Check sheet for the modelled part. Datum: model origin and axes. Units: mm. A direction names the side the tool comes from. Round coordinates to 2 decimals unless told otherwise and drop trailing zeros. Write each loop counter-clockwise with the first axis right and the second up, starting at its lowest first coordinate (ties: lowest second). Pieces come first, ordered by that corner, then holes. Notation, with made-up numbers: M 76.25,48 L 130.25,48 A29 ccw 130.25,72 Z; hole C 68.25,86 d1. An arc over 180 degrees is marked long. Answer in a Markdown table with one row per item.
```python
from build123d import *

# Parameters (mm, degrees)
BASPROSKE_W             = 19.05
BASPROSKE_H             = 19.957142857
TOOTHCUT_DEPTH          = 35.051102802
TEETHCUTS_COUNT         = 20
BORSKE_R                = 6.35
BORE_DEPTH              = 50.8000508
KEYSKE_W                = 3.175
KEYSKE_H                = 7.4676
KEYWAY_DEPTH            = 50.8000508
SKETCH1_W               = 3.175
SKETCH1_H               = 0.4064
CUT_EXTRUDE4_DEPTH      = 34.838053031
CUT_EXTRUDE4_DEPTH_BACK = 34.838053031


with BuildPart() as part:
    # BasProSke → Base-Revolve (revolve)
    with BuildSketch(Plane(origin=(0, 0, 0), x_dir=(1, 0, 0), z_dir=(0, 1, 0)), mode=Mode.PRIVATE) as base_revolve_sk:
        with Locations((9.525, 9.978571429)):
            Rectangle(BASPROSKE_W, BASPROSKE_H)
    revolve(base_revolve_sk.sketch.rotate(Axis((-10, 0, 0), (1, 0, 0)), 180), axis=Axis((-10, 0, 0), (1, 0, 0)))

    # TooCutSke → ToothCut (cut, through all)
    with BuildSketch(Plane(origin=(0, 0, 0), x_dir=(0, 0, -1), z_dir=(1, 0, 0))):
        with BuildLine():
            ThreePointArc((0.93220263, 15.846334036), (0, 15.87373), (-0.93220263, 15.846334036))
            ThreePointArc((-0.93220263, 15.846334036), (-1.519014467, 17.957902446), (-2.709431151, 19.798004997))
            ThreePointArc((-2.709431151, 19.798004997), (0, 19.982542857), (2.709431151, 19.798004997))
            ThreePointArc((2.709431151, 19.798004997), (1.519014467, 17.957902446), (0.93220263, 15.846334036))
        make_face()
    toothcut = extrude(amount=TOOTHCUT_DEPTH, mode=Mode.SUBTRACT)

    # TeethCuts: ToothCut ×20 about axis
    teethcuts_axis = Axis((0, 0, 0), (1, 0, 0))
    for i in range(1, TEETHCUTS_COUNT):
        add(toothcut.rotate(teethcuts_axis, i * 360 / TEETHCUTS_COUNT), mode=Mode.SUBTRACT)

    # BorSke → Bore (cut, symmetric)
    with BuildSketch(Plane(origin=(0, 0, 0), x_dir=(0, 0, -1), z_dir=(1, 0, 0))):
        with Locations(Location((0, 0, 0), (0, 0, 180))):
            Circle(BORSKE_R)
    extrude(amount=BORE_DEPTH, both=True, mode=Mode.SUBTRACT)

    # KeySke → Keyway (cut, symmetric)
    with BuildSketch(Plane(origin=(0, 0, 0), x_dir=(0, 0, -1), z_dir=(1, 0, 0))):
        with Locations((0, 3.7338)):
            Rectangle(KEYSKE_W, KEYSKE_H)
    extrude(amount=KEYWAY_DEPTH, both=True, mode=Mode.SUBTRACT)

    # Sketch1 → Cut-Extrude4 (cut, two sides)
    with BuildSketch(Plane(origin=(19.05, 0, 0), x_dir=(0, 0, -1), z_dir=(1, 0, 0))) as cut_extrude4_sk:
        with Locations((0, 7.6708)):
            Rectangle(SKETCH1_W, SKETCH1_H)
    extrude(amount=CUT_EXTRUDE4_DEPTH, mode=Mode.SUBTRACT)
    extrude(cut_extrude4_sk.sketch, amount=-CUT_EXTRUDE4_DEPTH_BACK, mode=Mode.SUBTRACT)


solid = part.part
```
1. Section check C-C, the plane y = 17. Record the cut outline in (x, z).
Found:
| item | result |
|---|---|
| outline | M 0,-9.48 L 19.05,-9.48 L 19.05,-7.38 L 0,-7.38 Z; M 0,-4.14 L 19.05,-4.14 L 19.05,-1.17 L 0,-1.17 Z; M 0,1.17 L 19.05,1.17 L 19.05,4.14 L 0,4.14 Z; M 0,7.38 L 19.05,7.38 L 19.05,9.48 L 0,9.48 Z |
2. Draft check along Y on faces 4 (the face through (9.39, -4.11, -17.5)), 5 (the face through (9.392, 7.004, 16.621)), 6 (the face through (9.39, 13.61, 11.74)). Enter one of: +Y half, -Y half, draft (parallel to the pull), parting line (faces both ways), or undercut.
Found:
| item | result |
|---|---|
| face 4 | undercut |
| face 5 | undercut |
| face 6 | +Y half |
3. Section check A-A, the plane z = 0. Record the cut outline in (x, y).
Found:
| item | result |
|---|---|
| outline | M 0,-15.87 L 19.05,-15.87 L 19.05,-6.35 L 0,-6.35 Z; M 0,7.87 L 19.05,7.87 L 19.05,15.87 L 0,15.87 Z |
4. Section check B-B, the plane y = 0. Record the cut outline in (x, z), and give its area (3 significant figures).
Found:
| item | result |
|---|---|
| outline | M 0,-15.87 L 19.05,-15.87 L 19.05,-6.35 L 0,-6.35 Z; M 0,6.35 L 19.05,6.35 L 19.05,15.87 L 0,15.87 Z |
| area | 363 mm2 |
5. Scan lines: L1, parallel to Z at x = 6.5, y = 0; L2, parallel to Y at x = 6, z = 17; L3, parallel to Z at x = 7, y = -15.5. Record each from-to range of solid material in increasing order.
Found:
| item | result |
|---|---|
| L1 | z = -15.87 to -6.35, 6.35 to 15.87 |
| L2 | y = -9.48 to -7.38, -4.14 to -1.17, 1.17 to 4.14, 7.38 to 9.48 |
| L3 | z = -9.34 to -6.17, -4.04 to 4.04, 6.17 to 9.34 |
6. Access from +Z, -Z, +X, -X, +Y, -Y to the whole of each face (thin tool, end or side, straight path). Record for faces 1 (the face through (9.392, 12.834, -9.341)), 2 (the face through (9.392, -6.963, 16.576)), 3 (the face through (9.392, 16.621, -7.004)).
Found:
| item | result |
|---|---|
| face 1 | +X, -X |
| face 2 | +Z, +X, -X |
| face 3 | +X, -X, +Y |
7. Go/stop test with flat-tipped pins: pin 1 (1.5 mm diameter, centred on x = 13, y = -11.5, fed in from +Z); pin 2 (1.9 mm diameter, centred on x = 14, y = 7, fed in from -Z); pin 3 (3 mm diameter, centred on x = 4, z = -14, fed in from -Y). Record where each tip stops, or that it passes through.
Found:
| item | result |
|---|---|
| pin 1 | stops at z = 13.88 |
| pin 2 | stops at z = -17.49 |
| pin 3 | stops at y = -14.42 |
